```python
from build123d import *

# Parameters (mm, degrees)
SKETCH1_R           = 12.5
SKETCH1_R_2         = 2.55
BOSS_EXTRUDE1_DEPTH = 3
SKETCH2_W           = 5.1
SKETCH2_H           = 5.1
CUT_EXTRUDE1_DEPTH  = 4


with BuildPart() as part:
    # Sketch1 → Boss-Extrude1 (new body)
    with BuildSketch(Plane(origin=(0, 0, 0), x_dir=(1, 0, 0), z_dir=(0, 1, 0))):
        with BuildLine():
            Line((15.75, -60.75), (-15.75, -60.75))
            ThreePointArc((-15.75, -60.75), (-18.578427125, -59.578427125), (-19.75, -56.75))
            Line((-19.75, -56.75), (-19.75, 17.25))
            ThreePointArc((-19.75, 17.25), (-18.578427125, 20.078427125), (-15.75, 21.25))
            Line((-15.75, 21.25), (15.75, 21.25))
            ThreePointArc((15.75, 21.25), (18.578427125, 20.078427125), (19.75, 17.25))
            Line((19.75, 17.25), (19.75, -56.75))
            ThreePointArc((19.75, -56.75), (18.578427125, -59.578427125), (15.75, -60.75))
        make_face()
        Circle(SKETCH1_R, mode=Mode.SUBTRACT)
        with Locations((10, -52.55)):
            Circle(SKETCH1_R_2, mode=Mode.SUBTRACT)
        with Locations((10, -32.55)):
            Circle(SKETCH1_R_2, mode=Mode.SUBTRACT)
        with Locations((0, -52.55)):
            Circle(SKETCH1_R_2, mode=Mode.SUBTRACT)
        with Locations((0, -32.55)):
            Circle(SKETCH1_R_2, mode=Mode.SUBTRACT)
        with Locations((-10, -52.55)):
            Circle(SKETCH1_R_2, mode=Mode.SUBTRACT)
        with Locations((-10, -32.55)):
            Circle(SKETCH1_R_2, mode=Mode.SUBTRACT)
        with BuildLine():
            Line((11.903984489, 14.096015511), (14.403984489, 16.596015511))
            ThreePointArc((14.403984489, 16.596015511), (16.596015511, 16.596015511), (16.596015511, 14.403984489))
            Line((16.596015511, 14.403984489), (14.096015511, 11.903984489))
            ThreePointArc((14.096015511, 11.903984489), (11.903984489, 11.903984489), (11.903984489, 14.096015511))
        make_face(mode=Mode.SUBTRACT)
        with BuildLine():
            Line((-11.903984489, 14.096015511), (-14.403984489, 16.596015511))
            ThreePointArc((-14.403984489, 16.596015511), (-16.596015511, 16.596015511), (-16.596015511, 14.403984489))
            Line((-16.596015511, 14.403984489), (-14.096015511, 11.903984489))
            ThreePointArc((-14.096015511, 11.903984489), (-11.903984489, 11.903984489), (-11.903984489, 14.096015511))
        make_face(mode=Mode.SUBTRACT)
        with BuildLine():
            Line((-11.903984489, -14.096015511), (-14.403984489, -16.596015511))
            ThreePointArc((-14.403984489, -16.596015511), (-16.596015511, -16.596015511), (-16.596015511, -14.403984489))
            Line((-16.596015511, -14.403984489), (-14.096015511, -11.903984489))
            ThreePointArc((-14.096015511, -11.903984489), (-11.903984489, -11.903984489), (-11.903984489, -14.096015511))
        make_face(mode=Mode.SUBTRACT)
        with BuildLine():
            Line((11.903984489, -14.096015511), (14.403984489, -16.596015511))
            ThreePointArc((14.403984489, -16.596015511), (16.596015511, -16.596015511), (16.596015511, -14.403984489))
            Line((16.596015511, -14.403984489), (14.096015511, -11.903984489))
            ThreePointArc((14.096015511, -11.903984489), (11.903984489, -11.903984489), (11.903984489, -14.096015511))
        make_face(mode=Mode.SUBTRACT)
    extrude(amount=BOSS_EXTRUDE1_DEPTH)

    # Sketch2 → Cut-Extrude1 (cut, through all)
    with BuildSketch(Plane(origin=(0, 3, 0), x_dir=(1, 0, 0), z_dir=(0, 1, 0))):
        with Locations((0, -32.55)):
            Rectangle(SKETCH2_W, SKETCH2_H)
    extrude(amount=-CUT_EXTRUDE1_DEPTH, mode=Mode.SUBTRACT)


solid = part.part
```
The model under review builds one solid part; all positions refer to its coordinate system, in mm. A direction names the side the tool comes from. Round coordinates to 2 decimals unless told otherwise and drop trailing zeros. Loops run counter-clockwise (first coordinate to the right, second up) from the corner with the lowest first, then second, coordinate; pieces in that order, holes last. Notation, with made-up numbers: (25, 67.5) - (77, 67.5) arc R20 ccw to (77, 85.5) - close; hole circle Ø5 at (56.5, 88.25). An arc over 180 degrees is marked (long way). Write each question's results on one line, items separated by ' | '. Start each with the question number.
Q1. Take a section at A-A on z = 52.55. Give the boundary of the cut face in (x, y).
Q2. Insertion check: P1, Ø6, axis at x = -2, z = 11, coming from the -Y side. The pin has a flat end and moves straight along its axis. Give the tip position at first contact, or say it passes through.
Q3. Draft analysis for pull direction X (two halves, no side actions). For faces 1 (the cylindrical face through (18.547, 1.479, -20.109)), 2 (the flat face through (0, 1, -21.25)), 3 (the cylindrical face through (-10.55, 1.48, 55.04)), 4 (the cylindrical face through (16.57, 1.48, 16.62)), state which applies: pulls with the +X half, pulls with the -X half, needs draft (parallel to the pull), parting line crosses it, or undercut.
Q4. Take a section at C-C on z = 0. Give the boundary of the cut face in (x, y).
Q5. Take a section at D-D on y = 1.2. Give the number of separate pieces and of enclosed holes in the cut face, plus the area to 3 significant figures.
Q6. Take a section at B-B on x = 0. Give the boundary of the cut face in (y, z).
Q7. Wall thickness on line 1 along X through (y, z) = (0.7, 52.55); line 2 along Z through (x, y) = (0, 0.65): over which ranges is each line inside the solid? List them lowest first. Write a range as [from, to].
Q8. Tool access review of faces 5 (the flat face through (0, 2, 35.1)), 6 (the flat face through (-19.75, 1, 20)): name each direction out of +Z, -Z, +X, -X, +Y, -Y from which nothing blocks a thin tool from reaching the whole face with its end or side.
Data:
1) outline: (-19.75, 0) - (-12.55, 0) - (-12.55, 3) - (-19.75, 3) - close; (-7.45, 0) - (-2.55, 0) - (-2.55, 3) - (-7.45, 3) - close; (2.55, 0) - (7.45, 0) - (7.45, 3) - (2.55, 3) - close; (12.55, 0) - (19.75, 0) - (19.75, 3) - (12.55, 3) - close
2) P1: stops at y = 0
3) face 1: pulls with the +X half | face 2: needs draft | face 3: undercut | face 4: undercut
4) outline: (-19.75, 0) - (-12.5, 0) - (-12.5, 3) - (-19.75, 3) - close; (12.5, 0) - (19.75, 0) - (19.75, 3) - (12.5, 3) - close
5) separate pieces: 1 | enclosed holes: 11 | area: 2,530 mm²
6) outline: (0, -21.25) - (3, -21.25) - (3, -12.5) - (0, -12.5) - close; (0, 12.5) - (3, 12.5) - (3, 30) - (0, 30) - close; (0, 35.1) - (3, 35.1) - (3, 50) - (0, 50) - close; (0, 55.1) - (3, 55.1) - (3, 60.75) - (0, 60.75) - close
7) line 1: x = [-19.75, -12.55], [-7.45, -2.55], [2.55, 7.45], [12.55, 19.75] | line 2: z = [-21.25, -12.5], [12.5, 30], [35.1, 50], [55.1, 60.75]
8) face 5: +Y, -Y | face 6: +Z, -Z, -X, +Y, -Y
